Verification items for the finished model (mm, model axes). A direction names the side the tool comes from. Coordinates: 2 decimals unless noted, no trailing zeros. Loops run counter-clockwise (first coordinate to the right, second up) from the corner with the lowest first, then second, coordinate; pieces in that order, holes last.
Q1. Access from +Z, -Z, +X, -X, +Y, -Y to the whole of each face (thin tool, end or side, straight path). Record for faces 1 (the face through (235, 236, 134.4)), 2 (the face through (201.6, 235, 100)), 3 (the face through (235, 67.2, 33)), 4 (the face through (33, 101, 67.2)).
Q2. Go/stop test with flat-tipped pins: P1, Ø4, axis at x = 155.5, y = 272.5, coming from the +Z side; P2, Ø1, axis at x = 241, z = 159.5, coming from the -Y side; P3, Ø3, axis at x = 276, z = 90, coming from the -Y side. Record where each tip stops, or that it passes through.
Q3. Sectioned sample at C-C (x = 219.5). Enter the section's corners in (y, z).
Q4. Sectioned sample at A-A (y = 95.5). Enter the section's corners in (x, z), then the cut area to 3 significant figures.
Q5. Sectioned sample at B-B (z = 172). Enter the section's corners in (x, y).
Q6. Mould release check, pull along X, two halves, no side actions. Record for faces 5 (the face through (166, 336, 99)), 6 (the face through (268.8, 168, 100)), 7 (the face through (0, 230, 77)): +X half, -X half, draft (parallel to the pull), parting line (faces both ways), or undercut.
Q7. Sectioned sample at D-D (z = 61.5). Enter the section's corners in (x, y).
Q8. Material ranges on probe 1 along X at (y, z) = (237, 73); probe 2 along Y at (x, z) = (294, 164.5); probe 3 along Y at (x, z) = (35.5, 92), recorded low to high.
```python
from build123d import *

# Parameters (mm, degrees)
F0_W     = 67.2
F0_H     = 67.2
F1_DEPTH = 201.6
F2_DEPTH = 134.4
F3_DEPTH = 67.2


with BuildPart() as f1:
    # F0 (on Top) → F1 (new body)
    with BuildSketch(Plane.XY):
        with Locations((33.6, 302.4)):
            Rectangle(F0_W, F0_H)
        with Locations((302.4, 302.4)):
            Rectangle(F0_W, F0_H)
        with Locations((302.4, 235.2)):
            Rectangle(F0_W, F0_H)
        with Locations((100.8, 302.4)):
            Rectangle(F0_W, F0_H)
        with Locations((235.2, 302.4)):
            Rectangle(F0_W, F0_H)
    extrude(amount=F1_DEPTH)



with BuildPart() as f2:
    # F0 (on Top) → F2 (new body)
    with BuildSketch(Plane.XY):
        with Locations((33.6, 235.2)):
            Rectangle(F0_W, F0_H)
        with Locations((33.6, 168)):
            Rectangle(F0_W, F0_H)
        with Locations((235.2, 235.2)):
            Rectangle(F0_W, F0_H)
        with Locations((302.4, 168)):
            Rectangle(F0_W, F0_H)
        with Locations((168, 302.4)):
            Rectangle(F0_W, F0_H)
    extrude(amount=F2_DEPTH)


with BuildPart() as f1_1:
    add(f1.part)

    add(f2.part)  # F3 merges F2
    # F0 (on Top) → F3 (join)
    with BuildSketch(Plane.XY):
        with Locations((100.8, 168)):
            Rectangle(F0_W, F0_H)
        with Locations((33.6, 100.8)):
            Rectangle(F0_W, F0_H)
        with Locations((235.2, 100.8)):
            Rectangle(F0_W, F0_H)
        with Locations((302.4, 100.8)):
            Rectangle(F0_W, F0_H)
        with Locations((235.2, 168)):
            Rectangle(F0_W, F0_H)
        with Locations((100.8, 235.2)):
            Rectangle(F0_W, F0_H)
        with Locations((168, 235.2)):
            Rectangle(F0_W, F0_H)
        with Locations((302.4, 33.6)):
            Rectangle(F0_W, F0_H)
    extrude(amount=F3_DEPTH)


solid = f1_1.part
```
Geometry check:
1. face 1: +Z, -X, -Y
1. face 2: +Z, -Y
1. face 3: +Z, -Z, -X, -Y
1. face 4: +Z, +X, -X, -Y
2. P1: stops at z = 134.4
2. P2: stops at y = 268.8
2. P3: stops at y = 134.4
3. outline: (67.2, 0) - (336, 0) - (336, 201.6) - (268.8, 201.6) - (268.8, 134.4) - (201.6, 134.4) - (201.6, 67.2) - (67.2, 67.2) - close
4. outline: (0, 0) - (67.2, 0) - (67.2, 67.2) - (0, 67.2) - close; (201.6, 0) - (336, 0) - (336, 67.2) - (201.6, 67.2) - close
4. area: 13,500 mm2
5. outline: (0, 268.8) - (134.4, 268.8) - (134.4, 336) - (0, 336) - close; (201.6, 268.8) - (268.8, 268.8) - (268.8, 201.6) - (336, 201.6) - (336, 336) - (201.6, 336) - close
6. face 5: draft
6. face 6: undercut
6. face 7: -X half
7. outline: (0, 67.2) - (67.2, 67.2) - (67.2, 134.4) - (134.4, 134.4) - (134.4, 201.6) - (201.6, 201.6) - (201.6, 67.2) - (268.8, 67.2) - (268.8, 0) - (336, 0) - (336, 336) - (0, 336) - close
8. probe 1: x = 0 to 67.2, 201.6 to 336
8. probe 2: y = 201.6 to 336
8. probe 3: y = 134.4 to 336
